from build123d import *

# Parameters (mm, degrees)
SKETCH_1_W          = 40
SKETCH_1_H          = 40
SKETCH_1_W_2        = 36
SKETCH_1_H_2        = 36
EXTRUDE_1_DEPTH     = 40
CUT_EXTRUDE_1_REACH = 62
SKETCH_2_R          = 10
SKETCH_2_R_2        = 1.6
CUT_EXTRUDE_2_REACH = 62
SKETCH_3_R          = 9.5
SKETCH_4_R          = 1.6
CUT_EXTRUDE_3_DEPTH = 61


with BuildPart() as part:
    # ｽｹｯﾁ1 → ﾎﾞｽ - 押し出し1 (new body)
    with BuildSketch(Plane(origin=(0, 0, 0), x_dir=(1, 0, 0), z_dir=(0, 1, 0))):
        Rectangle(SKETCH_1_W, SKETCH_1_H)
        Rectangle(SKETCH_1_W_2, SKETCH_1_H_2, mode=Mode.SUBTRACT)
    extrude(amount=EXTRUDE_1_DEPTH)

    # ｽｹｯﾁ2 → ｶｯﾄ - 押し出し1 (cut, up to next)
    with BuildSketch(Plane(origin=(0, 0, -20), x_dir=(-1, 0, 0), z_dir=(0, 0, -1)), mode=Mode.PRIVATE) as cut_extrude_1_sk1:
        with Locations((0, 20)):
            Circle(SKETCH_2_R)
    cut_extrude_1_tool1 = extrude(cut_extrude_1_sk1.sketch, amount=-CUT_EXTRUDE_1_REACH, mode=Mode.PRIVATE) & part.part
    # ｽｹｯﾁ2 → ｶｯﾄ - 押し出し1 (cut, up to next)
    with BuildSketch(Plane(origin=(0, 0, -20), x_dir=(-1, 0, 0), z_dir=(0, 0, -1)), mode=Mode.PRIVATE) as cut_extrude_1_sk2:
        with Locations((0, 33)):
            Circle(SKETCH_2_R_2)
    cut_extrude_1_tool2 = extrude(cut_extrude_1_sk2.sketch, amount=-CUT_EXTRUDE_1_REACH, mode=Mode.PRIVATE) & part.part
    # ｽｹｯﾁ2 → ｶｯﾄ - 押し出し1 (cut, up to next)
    with BuildSketch(Plane(origin=(0, 0, -20), x_dir=(-1, 0, 0), z_dir=(0, 0, -1)), mode=Mode.PRIVATE) as cut_extrude_1_sk3:
        with Locations((13, 20)):
            Circle(SKETCH_2_R_2)
    cut_extrude_1_tool3 = extrude(cut_extrude_1_sk3.sketch, amount=-CUT_EXTRUDE_1_REACH, mode=Mode.PRIVATE) & part.part
    # ｽｹｯﾁ2 → ｶｯﾄ - 押し出し1 (cut, up to next)
    with BuildSketch(Plane(origin=(0, 0, -20), x_dir=(-1, 0, 0), z_dir=(0, 0, -1)), mode=Mode.PRIVATE) as cut_extrude_1_sk4:
        with Locations((0, 7)):
            Circle(SKETCH_2_R_2)
    cut_extrude_1_tool4 = extrude(cut_extrude_1_sk4.sketch, amount=-CUT_EXTRUDE_1_REACH, mode=Mode.PRIVATE) & part.part
    # ｽｹｯﾁ2 → ｶｯﾄ - 押し出し1 (cut, up to next)
    with BuildSketch(Plane(origin=(0, 0, -20), x_dir=(-1, 0, 0), z_dir=(0, 0, -1)), mode=Mode.PRIVATE) as cut_extrude_1_sk5:
        with Locations((-13, 20)):
            Circle(SKETCH_2_R_2)
    cut_extrude_1_tool5 = extrude(cut_extrude_1_sk5.sketch, amount=-CUT_EXTRUDE_1_REACH, mode=Mode.PRIVATE) & part.part
    add(cut_extrude_1_tool1.solids().sort_by_distance((0, 20, -20))[0], mode=Mode.SUBTRACT)
    add(cut_extrude_1_tool2.solids().sort_by_distance((0, 33, -20))[0], mode=Mode.SUBTRACT)
    add(cut_extrude_1_tool3.solids().sort_by_distance((-13, 20, -20))[0], mode=Mode.SUBTRACT)
    add(cut_extrude_1_tool4.solids().sort_by_distance((0, 7, -20))[0], mode=Mode.SUBTRACT)
    add(cut_extrude_1_tool5.solids().sort_by_distance((13, 20, -20))[0], mode=Mode.SUBTRACT)

    # ｽｹｯﾁ3 → ｶｯﾄ - 押し出し2 (cut, up to next)
    with BuildSketch(Plane.XY.offset(20), mode=Mode.PRIVATE) as cut_extrude_2_sk1:
        with Locations((0, 20)):
            Circle(SKETCH_3_R)
    cut_extrude_2_tool1 = extrude(cut_extrude_2_sk1.sketch, amount=-CUT_EXTRUDE_2_REACH, mode=Mode.PRIVATE) & part.part
    add(cut_extrude_2_tool1.solids().sort_by_distance((0, 20, 20))[0], mode=Mode.SUBTRACT)

    # ｽｹｯﾁ4 → ｶｯﾄ - 押し出し3 (cut, through all)
    with BuildSketch(Plane.ZY.offset(20)):
        with Locations((15, 5)):
            Circle(SKETCH_4_R)
        with Locations((-15, 5)):
            Circle(SKETCH_4_R)
        with Locations((15, 35)):
            Circle(SKETCH_4_R)
        with Locations((-15, 35)):
            Circle(SKETCH_4_R)
    extrude(amount=-CUT_EXTRUDE_3_DEPTH, mode=Mode.SUBTRACT)


solid = part.part
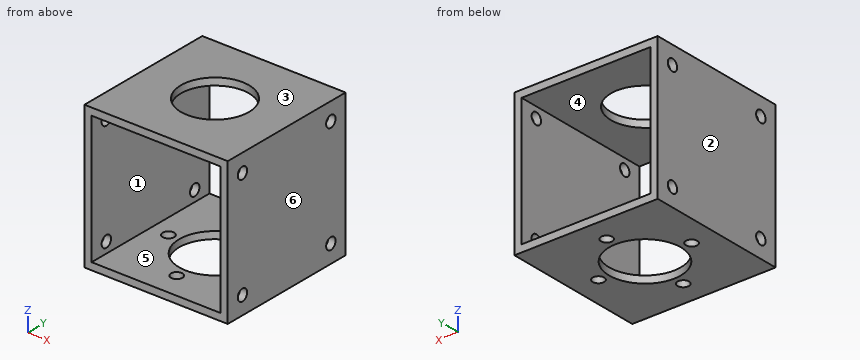
CAD build for the part. Positions are in the model's coordinates, mm. Face numbers are marked on the shaded views. A direction names the side the tool comes from. Coordinates: 2 decimals unless noted, no trailing zeros. Write each loop counter-clockwise with the first axis right and the second up, starting at its lowest first coordinate (ties: lowest second). Pieces come first, ordered by that corner, then holes. Notation, with made-up numbers: (-39, 19) - (-16, 19) arc R21 ccw to (-16, 33) - close; hole circle Ø2 at (68, 66.25). An arc over 180 degrees is marked (long way). Use a Markdown table: item, result. Add a question column.
Item 1: Band-saw the part on C-C, the plane y = 20. Give the cut face in (x, z).
Item 2: 3-axis set-ups, long thin cutter, end or side, ignore diameter. For the marked faces 5 and 6: which of +Z, -Z, +X, -X, +Y, -Y reach the whole face in a straight line?
Item 3: Flat gauge pin, fed straight in: pin 1 (2.5 mm diameter, centred on y = 5, z = -15, fed in from +X). Where does the tip first touch, or does it go through?
Item 4: Band-saw the part on D-D, the plane z = -15. Give the cut face in (x, y).
Item 5: Band-saw the part on A-A, the plane z = -5. Give the cut face in (x, y), and give its area (3 significant figures).
Item 6: Mould opens along X. For the marked faces 1, 2, 3 and 4 say: pulls with the +X half, pulls with the -X half, needs draft (parallel to the pull), parting line crosses it, or undercut.
Item 7: Drill centre lines: L1, parallel to Y at x = 19.2, z = 15; L2, parallel to X at y = 29, z = 5. Where is each one in solid material? Low to high. Write a range as from..to.
Item 8: Band-saw the part on B-B, the plane x = 0. Give the cut face in (y, z).
Numbers:
| question | item | result |
|---|---|---|
| 1 | outline | (-20, -20) - (-14.6, -20) - (-14.6, -18) - (-18, -18) - (-18, 18) - (-9.5, 18) - (-9.5, 20) - (-20, 20) - close; (-11.4, -20) - (-10, -20) - (-10, -18) - (-11.4, -18) - close; (9.5, 18) - (18, 18) - (18, -18) - (14.6, -18) - (14.6, -20) - (20, -20) - (20, 20) - (9.5, 20) - close; (10, -20) - (11.4, -20) - (11.4, -18) - (10, -18) - close |
| 2 | face 5 | +Y, -Y |
| 2 | face 6 | +Z, -Z, +X, +Y, -Y |
| 3 | pin 1 | through |
| 4 | outline | (-20, 0) - (-18, 0) - (-18, 3.4) - (-20, 3.4) - close; (-20, 6.6) - (-18, 6.6) - (-18, 33.4) - (-20, 33.4) - close; (-20, 36.6) - (-18, 36.6) - (-18, 40) - (-20, 40) - close; (18, 0) - (20, 0) - (20, 3.4) - (18, 3.4) - close; (18, 6.6) - (20, 6.6) - (20, 33.4) - (18, 33.4) - close; (18, 36.6) - (20, 36.6) - (20, 40) - (18, 40) - close |
| 5 | outline | (-20, 0) - (-18, 0) - (-18, 40) - (-20, 40) - close; (18, 0) - (20, 0) - (20, 40) - (18, 40) - close |
| 5 | area | 160 mm2 |
| 6 | face 1 | undercut |
| 6 | face 2 | pulls with the -X half |
| 6 | face 3 | needs draft |
| 6 | face 4 | undercut |
| 7 | L1 | 0..3.4, 6.6..33.4, 36.6..40 |
| 7 | L2 | -20..-18, 18..20 |
| 8 | outline | (0, -20) - (5.4, -20) - (5.4, -18) - (0, -18) - close; (0, 18) - (10.5, 18) - (10.5, 20) - (0, 20) - close; (8.6, -20) - (10, -20) - (10, -18) - (8.6, -18) - close; (29.5, 18) - (40, 18) - (40, 20) - (29.5, 20) - close; (30, -20) - (31.4, -20) - (31.4, -18) - (30, -18) - close; (34.6, -20) - (40, -20) - (40, -18) - (34.6, -18) - close |
